Could you check a few things on this model? Use its own coordinates, in mm. A direction names the side the tool comes from. Give positions to 0.01 mm unless a question says otherwise; leave off trailing zeros. Write each loop counter-clockwise with the first axis right and the second up, starting at its lowest first coordinate (ties: lowest second). Pieces come first, ordered by that corner, then holes. Notation, with made-up numbers: M 48.25,21 L 95.25,21 A19 ccw 95.25,39 Z; hole C -20,1.5 d11. An arc over 180 degrees is marked long. Use one line per item in the form item = value.
Autodesk Inventor part; units mm, degrees
ref_plane "Work Plane1" through (3.15, 0, 6.5) normal (0, 0, 1) x (1, 0, 0)
ref_plane "YZ Plane" through (0, 0, 0) normal (1, 0, 0) x (0, 1, 0)
ref_plane "XZ Plane" through (0, 0, 0) normal (0, 1, 0) x (-1, 0, 0)
sketch "Sketch1" plane through (0, 0, 0) normal (0, 0, 1) x (1, 0, 0)
  line L0 (0, 0) -> (17.5, 0)
  line L1 (0, 0) -> (0, 6.5)
  line L2 (0, 6.5) -> (6.3, 6.5)
  line L3 (6.3, 6.5) -> (6.3, 11)
  line L4 (6.3, 11) -> (7.658, 11)
  line L5 (7.658, 11) -> (7.9, 8.8125)
  line L6 (7.9, 8.8125) -> (15.9, 8.8125)
  line L7 (15.9, 8.8125) -> (16.142, 11)
  line L8 (16.142, 11) -> (17.5, 11)
  line L9 (17.5, 11) -> (17.5, 0)
  line L10 (7.658, 11) -> (16.142, 11) construction
  line L11 (11.9, 8.8125) -> (11.9, 11) construction
  dimension "d0" = 13
  dimension "d2" = 22
  dimension "d3" = 11.2
  dimension "d4" = 1.358
  dimension "d5" = 8
  dimension "d6" = 1.358
  dimension "d7" = 17.625
  dimension "d8" = 6.3
  dimension "d9" = 17.5
revolve "Revolution1" add sketch "Sketch1" angle 360 about axis through (0, 0, 0) along (1, 0, 0)
sketch "Sketch2" plane through (17.5, 0, 0) normal (1, 0, 0) x (0, 0, -1)
  circle A0 centre (0, 0) radius 11
hole "Hole1" at (17.5, 0, 0) direction (-1, 0, 0) diameter 5 end through all
ref_plane "Work Plane1" through (3.15, 0, 6.5) normal (0, 0, 1) x (1, 0, 0)
sketch "Sketch4" plane through (3.15, 0, 6.5) normal (0, 0, 1) x (1, 0, 0)
  line L0 (3.15, -6.5) -> (3.15, 6.5)
  line L1 (-3.15, -6.5) -> (-3.15, 6.5)
  line L2 (-3.15, 0) -> (3.15, 0) construction
  point P0 (0, 0)
hole "Hole2" at (3.15, 0, 6.5) direction (0, 0, -1) diameter 3 end up to surface
pattern_circular "Circular Pattern1" count 2 over 90 about axis through (-18.1966, 0, 0) along (-1, 0, 0) of "Hole2"
equation "\"d6\" = d4"
properties part number "GT2 Timing Pulley" material "Aluminum 6061"
1) I want a section at A-A, the plane y = 0. Please give me the cut outline in (x, z), plus the area to 3 significant figures.
Checked values:
outline = M 0,-6.5 L 6.3,-6.5 L 6.3,-11 L 7.66,-11 L 7.9,-8.81 L 15.9,-8.81 L 16.14,-11 L 17.5,-11 L 17.5,-2.5 L 0,-2.5 Z; M 0,2.5 L 1.65,2.5 L 1.65,6.5 L 0,6.5 Z; M 4.65,2.5 L 17.5,2.5 L 17.5,11 L 16.14,11 L 15.9,8.81 L 7.9,8.81 L 7.66,11 L 6.3,11 L 6.3,6.5 L 4.65,6.5 Z
area = 193 mm2
2) For faces 1 (the cylindrical face through (3.194, -1.409, -6.345)), 2 (the cylindrical face through (11.956, -6.993, -5.362)), 3 (the cylindrical face through (6.99, -2.38, -10.74)), 4 (the flat face through (0, 3, 0)), 5 (the cylindrical face through (4.614, 0.325, 4.219)), which set-ups out of +Z, -Z, +X, -X, +Y, -Y let a thin tool reach every point of the face, with its end or its side?
Checked values:
face_1 = -X
face_2 = none
face_3 = +X, -X
face_4 = +Z, -Z, -X, +Y, -Y
face_5 = +Z
3) If I drill on L1, parallel to Z at x = 10, y = 0; L2, parallel to Z at x = 6.25, y = 0; L3, parallel to X at y = -8.5, z = -6, over which ranges is the centre line in solid material (lowest first)?
Checked values:
L1 = -8.81 to -2.5, 2.5 to 8.81
L2 = -6.5 to -2.5, 2.5 to 6.5
L3 = 6.3 to 7.72, 16.08 to 17.5
4) For pin 1 Ø2 at (x, z) = (2, 2.5) entering from -Y; pin 2 Ø5 at (x, z) = (3.5, 7.5) entering from +Y; pin 3 Ø3.5 at (x, y) = (3.15, 0) entering from -Z, each with a flat end and sliding along its axis, tell me the tip position at first contact or that it passes through.
Checked values:
pin_1 = -6.32
pin_2 = 4.15
pin_3 = -6.5
5) Thinking about a two-plate mould opening in Z: for faces 6 (the cylindrical face through (4.614, 4.218, -0.325)), 7 (the cylindrical face through (16.83, -2.38, -10.74)), 8 (the flat face through (6.3, 5, -5)), 9 (the cylindrical face through (8.63, -2.11, -1.34)), which applies, released by +Z, released by -Z, zero draft, split by the parting line, or undercut?
Checked values:
face_6 = undercut
face_7 = split by the parting line
face_8 = zero draft
face_9 = undercut
6) I want a section at C-C, the plane x = 3.15. Please give me the cut outline in (y, z).
Checked values:
outline = M -1.5,2 L -1.5,6.32 A6.5 ccw long 6.32,-1.5 L 2,-1.5 A2.5 cw long Z; M 1.5,2 A2.5 cw 2,1.5 L 6.32,1.5 A6.5 ccw 1.5,6.32 Z
7) I want a section at D-D, the plane x = 13. Please give me the cut outline in (y, z) (1 decimal), plus the area to 3 significant figures.
Checked values:
outline = C 0,0 d17.6; hole C 0,0 d5
area = 224 mm2
